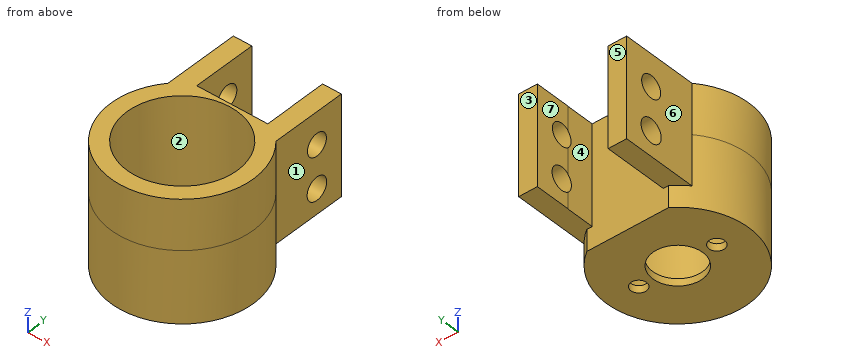
from build123d import *

# Parameters (mm, degrees)
SKETCH_1_R           = 14.75
EXTRUDE_1_DEPTH      = 1
SKETCH_2_R           = 1.5
CUT_EXTRUDE_1_DEPTH  = 1
SKETCH_3_R           = 1.1
CUT_EXTRUDE_2_DEPTH  = 1
SKETCH_4_R           = 3.5
CUT_EXTRUDE_3_DEPTH  = 4
SKETCH_5_OUTSIDE_W   = 39.846
SKETCH_5_OUTSIDE_H   = 39.846
SKETCH_5_OUTSIDE_R   = 7
CUT_EXTRUDE_4_DEPTH  = 10
SKETCH_6_R           = 8.75
SKETCH_6_R_2         = 6.75
EXTRUDE_1_2_DEPTH    = 10
SKETCH_7_W           = 20
SKETCH_7_H           = 5.176336695
EXTRUDE_2_DEPTH      = 9
CUT_EXTRUDE_5_DEPTH  = 2
SKETCH_9_W           = 10
SKETCH_9_H           = 4
CUT_EXTRUDE_6_DEPTH  = 12
CHAMFER_START        = 3
CHAMFER_2_DEPTH      = 7
SKETCH_10_W          = 5
SKETCH_10_H          = 7
SKETCH_10_W_2        = 5.030534445
EXTRUDE_3_DEPTH      = 5
SKETCH_11_W          = 0.39232609
SKETCH_11_H          = 7
CUT_EXTRUDE_7_DEPTH  = 22
SKETCH_12_W          = 2
SKETCH_12_H          = 7
CUT_EXTRUDE_8_DEPTH  = 12
SKETCH_13_R          = 1.65
CUT_EXTRUDE_9_DEPTH  = 10
SKETCH_14_R          = 1.6
CUT_EXTRUDE_10_DEPTH = 24
SKETCH_15_R          = 7.75
CUT_EXTRUDE_11_DEPTH = 9
SKETCH_16_R          = 7.75
EXTRUDE_4_DEPTH      = 10
SKETCH_17_W          = 18.442899184
SKETCH_17_H          = 2.260029227
CUT_EXTRUDE_12_DEPTH = 3
EXTRUDE_START        = 7
SKETCH_18_R          = 7.75
EXTRUDE_5_DEPTH      = 7
SKETCH_19_R          = 1.55
CUT_EXTRUDE_13_DEPTH = 17


with BuildPart() as part:
    # 草图1 → Extrude 1 (new body)
    with BuildSketch(Plane.XY):
        Circle(SKETCH_1_R)
    extrude(amount=EXTRUDE_1_DEPTH)

    # 草图2 → 切除-拉伸1 (cut)
    with BuildSketch(Plane.XY.offset(1)):
        with Locations((-11.5, 0)):
            Circle(SKETCH_2_R)
        with Locations((11.5, 0)):
            Circle(SKETCH_2_R)
        with Locations((0, -11.5)):
            Circle(SKETCH_2_R)
    extrude(amount=-CUT_EXTRUDE_1_DEPTH, mode=Mode.SUBTRACT)

    # 草图3 → 切除-拉伸2 (cut)
    with BuildSketch(Plane.XY.offset(1)):
        with Locations((-5.5, 0)):
            Circle(SKETCH_3_R)
        with Locations((5.5, 0)):
            Circle(SKETCH_3_R)
    extrude(amount=-CUT_EXTRUDE_2_DEPTH, mode=Mode.SUBTRACT)

    # 草图4 → 切除-拉伸3 (cut)
    with BuildSketch(Plane(origin=(0, 0, 0), x_dir=(-1, 0, 0), z_dir=(0, 0, -1))):
        Circle(SKETCH_4_R)
    extrude(amount=-CUT_EXTRUDE_3_DEPTH, mode=Mode.SUBTRACT)

    # 草图5 outside → 切除-拉伸4 (cut)
    with BuildSketch(Plane(origin=(0, 0, 0), x_dir=(-1, 0, 0), z_dir=(0, 0, -1))):
        Rectangle(SKETCH_5_OUTSIDE_W, SKETCH_5_OUTSIDE_H)
        Circle(SKETCH_5_OUTSIDE_R, mode=Mode.SUBTRACT)
    extrude(amount=-CUT_EXTRUDE_4_DEPTH, mode=Mode.SUBTRACT)

    # 草图6 → Extrude 1 2 (add)
    with BuildSketch(Plane(origin=(0, 0, 0), x_dir=(-1, 0, 0), z_dir=(0, 0, -1))):
        Circle(SKETCH_6_R)
        Circle(SKETCH_6_R_2, mode=Mode.SUBTRACT)
    extrude(amount=-EXTRUDE_1_2_DEPTH)

    # 草图7 → 凸台-拉伸2 (add)
    with BuildSketch(Plane.XY.offset(1)):
        with Locations((0, 9.588168348)):
            Rectangle(SKETCH_7_W, SKETCH_7_H)
    extrude(amount=EXTRUDE_2_DEPTH)

    # 草图8 → 切除-拉伸5 (cut)
    with BuildSketch(Plane(origin=(0, 0, 1), x_dir=(-1, 0, 0), z_dir=(0, 0, -1))):
        with BuildLine():
            Line((5.25, 7), (10, 7))
            Line((10, 7), (10, 12.176336695))
            Line((10, 12.176336695), (-10, 12.176336695))
            Line((-10, 12.176336695), (-10, 7))
            Line((-10, 7), (-5.25, 7))
            ThreePointArc((-5.25, 7), (0, 8.75), (5.25, 7))
        make_face()
    extrude(amount=-CUT_EXTRUDE_5_DEPTH, mode=Mode.SUBTRACT)

    # 草图9 → 切除-拉伸6 (cut)
    with BuildSketch(Plane.XY.offset(10)):
        with Locations((0, 10.176336695)):
            Rectangle(SKETCH_9_W, SKETCH_9_H)
    extrude(amount=-CUT_EXTRUDE_6_DEPTH, mode=Mode.SUBTRACT)

    # 倒角1
    # the kernel refuses this chamfer: 5, 3.571428571 mm, written as the material it adds along each edge
    with BuildSketch(Plane(origin=(5.25, 7, 10), x_dir=(0.718685473033907, -0.6953353082146982, 0), z_dir=(0, 0, -1))) as chamfer_1_piece_1:
        with BuildLine():
            Line((2.129047938, 0.190960276), (3.191245845, -3.221004807))
            Line((3.191245845, -3.221004807), (3.121712315, -3.292873355))
            ThreePointArc((3.121712315, -3.292873355), (1.559431919, -1.647908743), (-0.069533531, -0.071868547))
            Line((-0.069533531, -0.071868547), (0.012505696, 0.099214956))
            ThreePointArc((0.012505696, 0.099214956), (1.064301984, 0.031360517), (2.116542242, 0.290175233))
            Line((2.116542242, 0.290175233), (2.129047938, 0.190960276))
        make_face()
    extrude(amount=7)

    # 倒角2: read off the stored shape, not the designer's step
    # 倒角2 outline → 倒角2 (add)
    with BuildSketch(Plane.XY.offset(CHAMFER_START)):
        with BuildLine():
            Line((-9.60767391, 7), (-6.822840892, 5.47826087))
            ThreePointArc((-6.822840892, 5.47826087), (-6.084183947, 6.288497889), (-5.25, 7))
            Line((-5.25, 7), (-9.60767391, 7))
        make_face()
    extrude(amount=CHAMFER_2_DEPTH)

    # 草图10 → 凸台-拉伸3 (add)
    with BuildSketch(Plane(origin=(0, 12.176336695, 0), x_dir=(1, 0, 0), z_dir=(0, 1, 0))):
        with Locations((-7.5, -6.5)):
            Rectangle(SKETCH_10_W, SKETCH_10_H)
        with Locations((7.484732777, -6.5)):
            Rectangle(SKETCH_10_W_2, SKETCH_10_H)
    extrude(amount=EXTRUDE_3_DEPTH)

    # 草图11 → 切除-拉伸7 (cut)
    with BuildSketch(Plane.XZ.offset(-7)):
        with Locations((-9.803836955, 6.5)):
            Rectangle(SKETCH_11_W, SKETCH_11_H)
        with Locations((9.803836955, 6.5)):
            Rectangle(SKETCH_11_W, SKETCH_11_H)
    extrude(amount=-CUT_EXTRUDE_7_DEPTH, mode=Mode.SUBTRACT)

    # 草图12 → 切除-拉伸8 (cut)
    with BuildSketch(Plane(origin=(0, 17.176336695, 0), x_dir=(1, 0, 0), z_dir=(0, 1, 0))):
        with Locations((-8.60767391, -6.5)):
            Rectangle(SKETCH_12_W, SKETCH_12_H)
        with Locations((8.60767391, -6.5)):
            Rectangle(SKETCH_12_W, SKETCH_12_H)
    extrude(amount=-CUT_EXTRUDE_8_DEPTH, mode=Mode.SUBTRACT)

    # 草图13 → 切除-拉伸9 (cut)
    with BuildSketch(Plane(origin=(-5, 0, 0), x_dir=(0, 0, -1), z_dir=(1, 0, 0))):
        with Locations(Location((-6.5, 13.176336695, 0), (0, 0, 90))):
            Circle(SKETCH_13_R)
    extrude(amount=-CUT_EXTRUDE_9_DEPTH, mode=Mode.SUBTRACT)

    # 草图14 → 切除-拉伸10 (cut)
    with BuildSketch(Plane(origin=(-5, 0, 0), x_dir=(0, 0, -1), z_dir=(1, 0, 0))):
        with Locations(Location((-6.5, 13.176336695, 0), (0, 0, 321.317812547))):
            Circle(SKETCH_14_R)
    extrude(amount=CUT_EXTRUDE_10_DEPTH, mode=Mode.SUBTRACT)

    # 倒角3
    # the kernel refuses this chamfer: 1, 0.862080288 mm, written as the material it adds along each edge
    with BuildSketch(Plane(origin=(-6.822840892, 5.47826087, 3), x_dir=(-0.8775324532256278, 0.47951725050910476, 0), z_dir=(0, 0, 1))) as chamfer_3_piece_1_section:
        with BuildLine():
            Line((0.991009207, -0.026752196), (0.072738558, 0.799334069))
            Line((0.072738558, 0.799334069), (0.052814761, 0.801078297))
            ThreePointArc((0.052814761, 0.801078297), (0.041497623, 0.398993566), (-0.019689565, 0.00351013))
            Line((-0.019689565, 0.00351013), (0, -0.02))
            ThreePointArc((0, -0.02), (0.495504604, -0.02), (0.991009207, -0.046752196))
            Line((0.991009207, -0.046752196), (0.991009207, -0.026752196))
        make_face()
    chamfer_3_piece_1 = extrude(amount=7, mode=Mode.PRIVATE)
    chamfer_3_piece_1 = split(chamfer_3_piece_1, bisect_by=Plane(origin=(-7.60767391, 5.47826087, 3), z_dir=(1, 0, 0)), keep=Keep.TOP, mode=Mode.PRIVATE)
    add(chamfer_3_piece_1)

    # 倒角4
    # the kernel refuses this chamfer: 1, 0.862080288 mm, written as the material it adds along each edge
    with BuildSketch(Plane(origin=(6.822840893, 5.47826087, 10), x_dir=(0.5907401034808368, -0.8068619027686523, 0), z_dir=(0, 0, -1))) as chamfer_4_piece_1_section:
        with BuildLine():
            Line((0.801958261, 0.032996956), (0.103787295, -0.985922474))
            Line((0.103787295, -0.985922474), (0.083960944, -0.988552263))
            ThreePointArc((0.083960944, -0.988552263), (0.045327257, -0.49383221), (-0.019826352, -0.002629788))
            Line((-0.019826352, -0.002629788), (0.000890684, 0.019980157))
            ThreePointArc((0.000890684, 0.019980157), (0.400985832, 0.011326106), (0.801067577, 0.052977113))
            Line((0.801067577, 0.052977113), (0.801958261, 0.032996956))
        make_face()
    chamfer_4_piece_1 = extrude(amount=7, mode=Mode.PRIVATE)
    chamfer_4_piece_1 = split(chamfer_4_piece_1, bisect_by=Plane(origin=(7.60767391, 5.47826087, 10), z_dir=(-1, 0, 0)), keep=Keep.TOP, mode=Mode.PRIVATE)
    add(chamfer_4_piece_1)

    # 草图15 → 切除-拉伸11 (cut)
    with BuildSketch(Plane.XY.offset(10)):
        Circle(SKETCH_15_R)
    extrude(amount=-CUT_EXTRUDE_11_DEPTH, mode=Mode.SUBTRACT)

    # 草图16 → 凸台-拉伸4 (add)
    with BuildSketch(Plane.XY.offset(10)):
        with BuildLine():
            Line((-5, 8.660254038), (-5, 8.176336695))
            Line((-5, 8.176336695), (5, 8.176336695))
            Line((5, 8.176336695), (5, 8.660254038))
            ThreePointArc((5, 8.660254038), (0, -10), (-5, 8.660254038))
        make_face()
        Circle(SKETCH_16_R, mode=Mode.SUBTRACT)
    extrude(amount=-EXTRUDE_4_DEPTH)

    # 草图17 → 切除-拉伸12 (cut)
    with BuildSketch(Plane(origin=(0, 0, 0), x_dir=(-1, 0, 0), z_dir=(0, 0, -1))):
        with Locations((-0.125316737, 9.306351309)):
            Rectangle(SKETCH_17_W, SKETCH_17_H)
    extrude(amount=-CUT_EXTRUDE_12_DEPTH, mode=Mode.SUBTRACT)

    # 草图18 → 凸台-拉伸5 (add)
    with BuildSketch(Plane.XY.offset(10).offset(EXTRUDE_START)):
        with BuildLine():
            Line((-5, 17.176336695), (-7.60767391, 17.176336695))
            Line((-7.60767391, 17.176336695), (-7.60767391, 6.49024635))
            ThreePointArc((-7.60767391, 6.49024635), (0, -10), (7.60767391, 6.49024635))
            Line((7.60767391, 6.49024635), (7.60767391, 17.176336695))
            Line((7.60767391, 17.176336695), (4.969465555, 17.176336695))
            Line((4.969465555, 17.176336695), (4.969465555, 12.176336695))
            Line((4.969465555, 12.176336695), (5, 12.176336695))
            Line((5, 12.176336695), (5, 8.176336695))
            Line((5, 8.176336695), (-5, 8.176336695))
            Line((-5, 8.176336695), (-5, 17.176336695))
        make_face()
        Circle(SKETCH_18_R, mode=Mode.SUBTRACT)
    extrude(amount=-EXTRUDE_5_DEPTH)

    # 草图19 → 切除-拉伸13 (cut)
    with BuildSketch(Plane(origin=(7.60767391, 0, 0), x_dir=(0, 0, -1), z_dir=(1, 0, 0))):
        with Locations((-12.5, 13.176336695)):
            Circle(SKETCH_19_R)
    extrude(amount=-CUT_EXTRUDE_13_DEPTH, mode=Mode.SUBTRACT)


solid = part.part
Could you check a few things on this model? Use its own coordinates, in mm. Face numbers are marked on the shaded views. A direction names the side the tool comes from. Coordinates: 2 decimals unless noted, no trailing zeros. Order: outer loops, then holes, each group sorted by start corner. A loop starts at its lowest first (then second) coordinate and runs counter-clockwise, first axis right, second up.
Q1. Which directions (+Z, -Z, +X, -X, +Y, -Y) give clear straight access to the entire face, cutting with the end or side of a thin tool? Please do the marked faces 4, 5, 6 and 7.
Q2. Thinking about a two-plate mould opening in X: for the marked faces 1, 2 and 3, which applies, released by +X, released by -X, zero draft, split by the parting line, or undercut?
Q3. Suppose I cut it at D-D on y = 13.5. Please give me the cut outline in (x, z).
Q4. Suppose I cut it at A-A on z = 6.5. Please give me the cut outline in (x, y), and give its area (3 significant figures).
Q5. Please list where these lines run through material, in increasing order: L1, parallel to Y at x = 6.75, z = 12.5; L2, parallel to X at y = 11, z = 16; L3, parallel to Y at x = 6.75, z = 11.5.
Q6. Suppose I cut it at B-B on x = -6.25. Please give me the cut outline in (y, z), and give its area (3 significant figures).
Q7. Will these pins go through, and if not, where does the flat tip stop? pin 1 (1.2 mm diameter, centred on y = 9.5, z = 9, fed in from -X); pin 2 (3 mm diameter, centred on y = 4, z = 5.5, fed in from -X); pin 3 (2 mm diameter, centred on x = 2.5, y = 4, fed in from -Z); pin 4 (0.8 mm diameter, centred on x = -6.5, y = 14, fed in from -Z).
Answer:
1. face 4: +Z, -Z
1. face 5: +Z, -Z, +X, -X, +Y
1. face 6: +Z, -Z, -X, +Y
1. face 7: +Z, -Z, +Y
2. face 1: released by +X
2. face 2: undercut
2. face 3: zero draft
3. outline: (-7.61, 3) - (-5, 3) - (-5, 4.88) - (-7.61, 4.88) - close; (-7.61, 8.12) - (-5, 8.12) - (-5, 10.98) - (-7.61, 10.98) - close; (-7.61, 14.02) - (-5, 14.02) - (-5, 17) - (-7.61, 17) - close; (4.97, 3) - (7.61, 3) - (7.61, 4.93) - (4.97, 4.93) - close; (4.97, 8.07) - (7.61, 8.07) - (7.61, 10.98) - (4.97, 10.98) - close; (4.97, 14.02) - (7.61, 14.02) - (7.61, 17) - (4.97, 17) - close
4. outline: (-7.61, 6.49) arc R10 ccw (long way) to (7.61, 6.49) - (7.61, 11.58) - (5, 11.58) - (5, 8.18) - (-5, 8.18) - (-5, 11.53) - (-7.61, 11.53) - close; (-7.61, 14.83) - (-5, 14.83) - (-5, 17.18) - (-7.61, 17.18) - close; (4.97, 14.78) - (7.61, 14.78) - (7.61, 17.18) - (4.97, 17.18) - close; hole circle Ø15.5 at (0, 0)
4. area: 144 mm2
5. L1: y = -7.38 to -3.81, 3.81 to 11.63, 14.73 to 17.18
5. L2: x = -7.61 to -5, 5 to 7.61
5. L3: y = -7.38 to -3.81, 3.81 to 11.99, 14.36 to 17.18
6. outline: (-7.81, 0) - (-0.8, 0) - (-0.8, 1) - (-4.58, 1) - (-4.58, 17) - (-7.81, 17) - close; (0.8, 0) - (7.81, 0) - (7.81, 3) - (17.18, 3) - (17.18, 17) - (4.58, 17) - (4.58, 1) - (0.8, 1) - close; hole circle Ø3.3 at (13.18, 6.5); hole circle Ø3.1 at (13.18, 12.5)
6. area: 232 mm2
7. pin 1: stops at x = -7.61
7. pin 2: stops at x = -9.68
7. pin 3: stops at z = 0
7. pin 4: stops at z = 3
